For this review, take the finished solid that the model builds, in its own axes (mm). A direction names the side the tool comes from. Coordinates: 2 decimals unless noted, no trailing zeros. Loops run counter-clockwise (first coordinate to the right, second up) from the corner with the lowest first, then second, coordinate; pieces in that order, holes last. Notation, with made-up numbers: (84.25, -37) -> (108.25, -37) arc R13 cw to (108.25, -22) -> close; hole circle Ø11 at (3.25, -30). An arc over 180 degrees is marked (long way). Use a Markdown table: item, result.
from build123d import *

# Parameters (mm, degrees)
BOSS_EXTRUDE1_DEPTH = 381
CUT_EXTRUDE1_DEPTH  = 382.531505268


with BuildPart() as part:
    # Sketch1 → Boss-Extrude1 (new body)
    with BuildSketch(Plane(origin=(0, 0, 0), x_dir=(0, 0, -1), z_dir=(1, 0, 0))):
        Polygon((0, 12.954), (0, -12.954), (-8.89, -12.954), (-8.89, -17.526), (-7.874, -17.526), (-7.874, -13.97), (0, -13.97), (0, -15.494), (1.016, -15.494), (1.016, 15.494), (0, 15.494), (0, 13.97), (-7.874, 13.97), (-7.874, 17.526), (-8.89, 17.526), (-8.89, 12.954), align=None)
    extrude(amount=BOSS_EXTRUDE1_DEPTH)

    # Sketch2 → Cut-Extrude1 (cut, through all)
    with BuildSketch(Plane(origin=(0, 0, -1.016), x_dir=(-1, 0, 0), z_dir=(0, 0, -1))):
        with BuildLine():
            Line((-368.554, 4.826), (-353.314, 4.826))
            ThreePointArc((-353.314, 4.826), (-348.488, 0), (-353.314, -4.826))
            Line((-353.314, -4.826), (-368.554, -4.826))
            ThreePointArc((-368.554, -4.826), (-373.38, 0), (-368.554, 4.826))
        make_face()
        with BuildLine():
            Line((-342.763230769, 4.826), (-327.523230769, 4.826))
            ThreePointArc((-327.523230769, 4.826), (-322.697230769, 0), (-327.523230769, -4.826))
            Line((-327.523230769, -4.826), (-342.763230769, -4.826))
            ThreePointArc((-342.763230769, -4.826), (-347.589230769, 0), (-342.763230769, 4.826))
        make_face()
        with BuildLine():
            Line((-316.972461538, 4.826), (-301.732461538, 4.826))
            ThreePointArc((-301.732461538, 4.826), (-296.906461538, 0), (-301.732461538, -4.826))
            Line((-301.732461538, -4.826), (-316.972461538, -4.826))
            ThreePointArc((-316.972461538, -4.826), (-321.798461538, 0), (-316.972461538, 4.826))
        make_face()
        with BuildLine():
            Line((-291.181692308, 4.826), (-275.941692308, 4.826))
            ThreePointArc((-275.941692308, 4.826), (-271.115692308, 0), (-275.941692308, -4.826))
            Line((-275.941692308, -4.826), (-291.181692308, -4.826))
            ThreePointArc((-291.181692308, -4.826), (-296.007692308, 0), (-291.181692308, 4.826))
        make_face()
        with BuildLine():
            Line((-265.390923077, 4.826), (-250.150923077, 4.826))
            ThreePointArc((-250.150923077, 4.826), (-245.324923077, 0), (-250.150923077, -4.826))
            Line((-250.150923077, -4.826), (-265.390923077, -4.826))
            ThreePointArc((-265.390923077, -4.826), (-270.216923077, 0), (-265.390923077, 4.826))
        make_face()
        with BuildLine():
            Line((-239.600153846, 4.826), (-224.360153846, 4.826))
            ThreePointArc((-224.360153846, 4.826), (-219.534153846, 0), (-224.360153846, -4.826))
            Line((-224.360153846, -4.826), (-239.600153846, -4.826))
            ThreePointArc((-239.600153846, -4.826), (-244.426153846, 0), (-239.600153846, 4.826))
        make_face()
        with BuildLine():
            Line((-213.809384615, 4.826), (-198.569384615, 4.826))
            ThreePointArc((-198.569384615, 4.826), (-193.743384615, 0), (-198.569384615, -4.826))
            Line((-198.569384615, -4.826), (-213.809384615, -4.826))
            ThreePointArc((-213.809384615, -4.826), (-218.635384615, 0), (-213.809384615, 4.826))
        make_face()
        with BuildLine():
            Line((-188.018615385, 4.826), (-172.778615385, 4.826))
            ThreePointArc((-172.778615385, 4.826), (-167.952615385, 0), (-172.778615385, -4.826))
            Line((-172.778615385, -4.826), (-188.018615385, -4.826))
            ThreePointArc((-188.018615385, -4.826), (-192.844615385, 0), (-188.018615385, 4.826))
        make_face()
        with BuildLine():
            Line((-162.227846154, 4.826), (-146.987846154, 4.826))
            ThreePointArc((-146.987846154, 4.826), (-142.161846154, 0), (-146.987846154, -4.826))
            Line((-146.987846154, -4.826), (-162.227846154, -4.826))
            ThreePointArc((-162.227846154, -4.826), (-167.053846154, 0), (-162.227846154, 4.826))
        make_face()
        with BuildLine():
            Line((-136.437076923, 4.826), (-121.197076923, 4.826))
            ThreePointArc((-121.197076923, 4.826), (-116.371076923, 0), (-121.197076923, -4.826))
            Line((-121.197076923, -4.826), (-136.437076923, -4.826))
            ThreePointArc((-136.437076923, -4.826), (-141.263076923, 0), (-136.437076923, 4.826))
        make_face()
        with BuildLine():
            Line((-110.646307692, 4.826), (-95.406307692, 4.826))
            ThreePointArc((-95.406307692, 4.826), (-90.580307692, 0), (-95.406307692, -4.826))
            Line((-95.406307692, -4.826), (-110.646307692, -4.826))
            ThreePointArc((-110.646307692, -4.826), (-115.472307692, 0), (-110.646307692, 4.826))
        make_face()
        with BuildLine():
            Line((-84.855538462, 4.826), (-69.615538462, 4.826))
            ThreePointArc((-69.615538462, 4.826), (-64.789538462, 0), (-69.615538462, -4.826))
            Line((-69.615538462, -4.826), (-84.855538462, -4.826))
            ThreePointArc((-84.855538462, -4.826), (-89.681538462, 0), (-84.855538462, 4.826))
        make_face()
        with BuildLine():
            Line((-59.064769231, 4.826), (-43.824769231, 4.826))
            ThreePointArc((-43.824769231, 4.826), (-38.998769231, 0), (-43.824769231, -4.826))
            Line((-43.824769231, -4.826), (-59.064769231, -4.826))
            ThreePointArc((-59.064769231, -4.826), (-63.890769231, 0), (-59.064769231, 4.826))
        make_face()
        with BuildLine():
            Line((-33.274, 4.826), (-18.034, 4.826))
            ThreePointArc((-18.034, 4.826), (-13.208, 0), (-18.034, -4.826))
            Line((-18.034, -4.826), (-33.274, -4.826))
            ThreePointArc((-33.274, -4.826), (-38.1, 0), (-33.274, 4.826))
        make_face()
    extrude(amount=-CUT_EXTRUDE1_DEPTH, mode=Mode.SUBTRACT)


solid = part.part
(1) Take a section at C-C on y = 0. State how many separate pieces and enclosed holes the cut face has, plus the area to 3 significant figures.
Found:
| item | result |
|---|---|
| separate pieces | 15 |
| enclosed holes | 0 |
| area | 33.0 mm^2 |
(2) For line 1 along Y through (x, z) = (350.5, 1.75); line 2 along Y through (x, z) = (315, 8.5); line 3 along Z through (x, y) = (320, 9), list the stretches that pass through material, from the lowest coordinate up.
Found:
| item | result |
|---|---|
| line 1 | y = -13.97 to -12.95, 12.95 to 13.97 |
| line 2 | y = -17.53 to -12.95, 12.95 to 17.53 |
| line 3 | z = -1.02 to 0 |
(3) For pin 1 Ø1.1 at (x, z) = (26.5, -0.5) entering from +Y; pin 2 Ø4 at (x, z) = (116.5, 3.5) entering from -Y; pin 3 Ø6 at (x, y) = (146.5, 1.5) entering from +Z; pin 4 Ø5 at (x, y) = (99, -8) entering from +Z, all flat-tipped, find the tip position at first contact; note any pin that passes through.
Found:
| item | result |
|---|---|
| pin 1 | stops at y = 15.49 |
| pin 2 | stops at y = -13.97 |
| pin 3 | passes through |
| pin 4 | stops at z = 0 |
(4) Take a section at A-A on z = 3.75. Write out the cut boundary in (x, y).
Found:
| item | result |
|---|---|
| outline | (0, -13.97) -> (381, -13.97) -> (381, -12.95) -> (0, -12.95) -> close; (0, 12.95) -> (381, 12.95) -> (381, 13.97) -> (0, 13.97) -> close |
(5) For faces 1 (the face through (188, -12.954, 4)), 2 (the face through (188, -13.97, 4)), 3 (the face through (381, 1.4, -0.4)), 4 (the face through (188, 13.97, 4)), 5 (the face through (188, -7, -1.016)), list the 3-axis set-ups (+Z, -Z, +X, -X, +Y, -Y) from which the entire face can be reached by the end or side of a thin tool; tool diameter is ignored.
Found:
| item | result |
|---|---|
| face 1 | +Z, +X, -X |
| face 2 | +X, -X, -Y |
| face 3 | +Z, -Z, +X, +Y, -Y |
| face 4 | +X, -X, +Y |
| face 5 | -Z, +X, -X, +Y, -Y |
(6) Take a section at B-B on x = 29.5. Write out the cut boundary in (y, z), plus the area to 3 significant figures.
Found:
| item | result |
|---|---|
| outline | (-17.53, 7.87) -> (-13.97, 7.87) -> (-13.97, 0) -> (-15.49, 0) -> (-15.49, -1.02) -> (-4.83, -1.02) -> (-4.83, 0) -> (-12.95, 0) -> (-12.95, 8.89) -> (-17.53, 8.89) -> close; (4.83, -1.02) -> (15.49, -1.02) -> (15.49, 0) -> (13.97, 0) -> (13.97, 7.87) -> (17.53, 7.87) -> (17.53, 8.89) -> (12.95, 8.89) -> (12.95, 0) -> (4.83, 0) -> close |
| area | 47.0 mm^2 |
